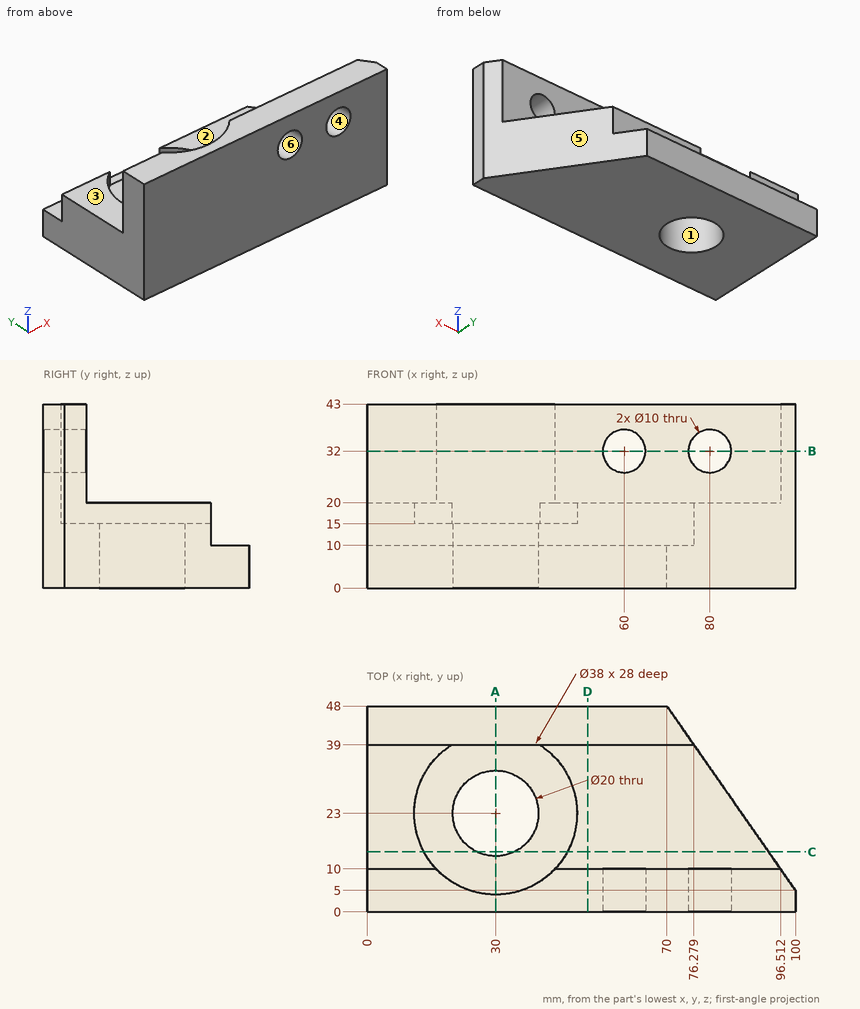
Job drawing, mm, ordinate dimensions from the low corner. One solid piece. A direction names the side the tool comes from. Give positions to 0.01 mm unless a question says otherwise; leave off trailing zeros. Loops run counter-clockwise (first coordinate to the right, second up) from the corner with the lowest first, then second, coordinate; pieces in that order, holes last. Notation, with made-up numbers: M 23.5,-1 L 46.5,-1 A28 cw 46.5,26 Z; hole C 86,-14 d9. An arc over 180 degrees is marked long. Answer in a Markdown table with one row per item. Add a question column.
Item 1: Band-saw the part on D-D on x = 51.5. Give the cut face in (y, z).
Item 2: Band-saw the part on B-B on z = 32. Give the cut face in (x, y).
Item 3: Drop flat-ended pins along their axis: P1, Ø21.5, axis at x = 13, y = 22, coming from the +Z side; P2, Ø3, axis at y = 22.5, z = 11.5, coming from the +X side; P3, Ø1, axis at x = 38.5, y = 31.5, coming from the +Z side; P4, Ø6, axis at x = 60, z = 32, coming from the +Y side. Give the stop position or say it passes through.
Item 4: Mould opens along Z. For the marked faces 3, 4, 5 and 6 say: +Z half, -Z half, draft (parallel to the pull), parting line (faces both ways), or undercut.
Item 5: Band-saw the part on C-C on y = 14. Give the cut face in (x, z).
Item 6: Band-saw the part on A-A on x = 30. Give the cut face in (y, z).
Item 7: Probe probe 1 along Z at (x, y) = (60, 5.5); probe 2 along Y at (x, z) = (7.5, 25.5); probe 3 along Y at (x, z) = (9.5, 17). List the from-to ranges inside material, lowest first.
Item 8: Tool access for the marked faces 1 and 2: list every direction of +Z, -Z, +X, -X, +Y, -Y with a clear straight run to the whole face (end or side of a thin tool).
Reply:
| question | item | result |
|---|---|---|
| 1 | outline | M 0,0 L 48,0 L 48,10 L 39,10 L 39,20 L 10,20 L 10,43 L 0,43 Z |
| 2 | outline | M 0,0 L 55,0 L 55,10 L 43.86,10 A19 cw 16.14,10 L 0,10 Z; M 65,0 L 75,0 L 75,10 L 65,10 Z; M 85,0 L 100,0 L 100,5 L 96.51,10 L 85,10 Z |
| 3 | P1 | stops at z = 20 |
| 3 | P2 | stops at x = 88.84 |
| 3 | P3 | stops at z = 15 |
| 3 | P4 | passes through |
| 4 | face 3 | +Z half |
| 4 | face 4 | undercut |
| 4 | face 5 | draft |
| 4 | face 6 | undercut |
| 5 | outline | M 0,0 L 25.64,0 L 25.64,15 L 13.27,15 L 13.27,20 L 0,20 Z; M 34.36,0 L 93.72,0 L 93.72,20 L 46.73,20 L 46.73,15 L 34.36,15 Z |
| 6 | outline | M 0,0 L 13,0 L 13,15 L 4,15 L 4,43 L 0,43 Z; M 33,0 L 48,0 L 48,10 L 39,10 L 39,15 L 33,15 Z |
| 7 | probe 1 | z = 0 to 27, 37 to 43 |
| 7 | probe 2 | y = 0 to 10 |
| 7 | probe 3 | y = 0 to 39 |
| 8 | face 1 | +Z, -Z |
| 8 | face 2 | +Z, +X, -X, +Y |
